Can you work these out from the drawing? Everything is in mm from the part's minimum corner. A direction names the side the tool comes from. Coordinates: 2 decimals unless noted, no trailing zeros. Loops run counter-clockwise (first coordinate to the right, second up) from the corner with the lowest first, then second, coordinate; pieces in that order, holes last.
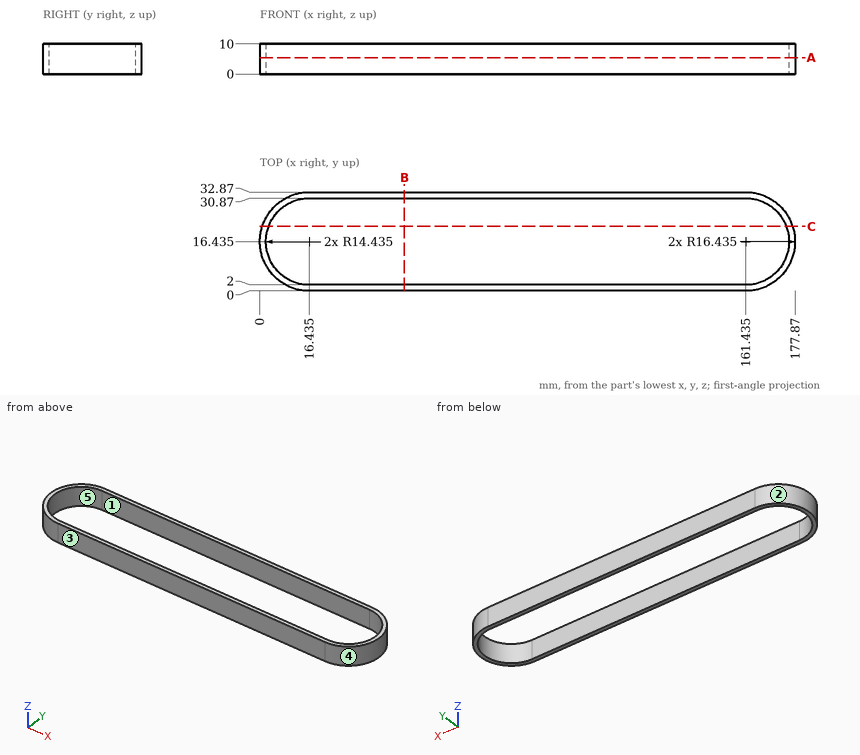
Item 1: I need wall thicknesses on line 1 along Y through (x, z) = (67, 5.75); line 2 along X through (y, z) = (17, 7.25); line 3 along X through (y, z) = (22, 7.5). Which ranges of each line are inside material? Lowest first, please.
Results are:
line 1: y = 0 to 2, 30.87 to 32.87
line 2: x = 0.01 to 2.01, 175.86 to 177.86
line 3: x = 0.97 to 3.12, 174.75 to 176.9
Item 2: On a 3-axis mill with a long thin cutter (end or side, diameter ignored), from which of +Z, -Z, +X, -X, +Y, -Y can I reach the whole of each face in a straight line? I mean the marked faces 1 and 2. Say none if no direction works.
Results are:
face 1: +Z, -Z
face 2: +Z, -Z, -X
Item 3: Suppose I cut it at A-A, the plane z = 5.5. Please give me the cut outline in (x, y) (3 decimals).
Results are:
outline: (16.435, 0) - (161.435, 0) arc R16.435 ccw to (161.435, 32.87) - (16.435, 32.87) arc R16.435 ccw to start; hole (16.435, 2) - (161.435, 2) arc R14.435 ccw to (161.435, 30.87) - (16.435, 30.87) arc R14.435 ccw to start
Item 4: We'd pull the mould along Y, two halves only. Please class the marked faces 3, 4 and 5: +Y half, -Y half, draft (parallel to the pull), parting line (faces both ways), or undercut.
Results are:
face 3: -Y half
face 4: parting line
face 5: undercut
Item 5: I'm going to push flat-ended pins straight in: P1, Ø3, axis at x = 117, z = 3, coming from the -Y side; P2, Ø2, axis at y = 13, z = 5.5, coming from the +X side; P3, Ø6, axis at y = 29, z = 5, coming from the -X side. Where does each tip first touch, or does it pass through?
Results are:
P1: stops at y = 0
P2: stops at x = 177.69
P3: stops at x = 3.07
Item 6: Suppose I cut it at C-C, the plane y = 21.5. Please give me the cut outline in (x, z).
Results are:
outline: (0.8, 0) - (2.92, 0) - (2.92, 10) - (0.8, 10) - close; (174.95, 0) - (177.07, 0) - (177.07, 10) - (174.95, 10) - close
Item 7: Suppose I cut it at B-B, the plane x = 48. Please give me the cut outline in (y, z), plus the area to 3 significant figures.
Results are:
outline: (0, 0) - (2, 0) - (2, 10) - (0, 10) - close; (30.87, 0) - (32.87, 0) - (32.87, 10) - (30.87, 10) - close
area: 40.0 mm2
